Autodesk Inventor part; units mm, degrees
ref_plane "YZ Plane" through (0, 0, 0) normal (1, 0, 0) x (0, 1, 0)
ref_plane "XZ Plane" through (0, 0, 0) normal (0, 1, 0) x (-1, 0, 0)
ref_plane "XY Plane" through (0, 0, 0) normal (0, 0, 1) x (1, 0, 0)
sketch "Sketch1" plane through (0, 0, 0) normal (0, 0, 1) x (1, 0, 0)
  line L0 (-320.04, 0) -> (320.04, 0)
  line L1 (0, -340.36) -> (0, 86.36)
  line L2 (-228.6, 25.4) -> (228.6, 25.4)
  line L3 (-76.2, -279.4) -> (76.2, -279.4)
  line L4 (-228.6, 0) -> (-76.2, -279.4)
  line L5 (228.6, 0) -> (76.2, -279.4)
  line L6 (228.6, 0) -> (228.6, 25.4)
  line L7 (-228.6, 0) -> (-228.6, 25.4)
  point P0 (0, 0)
  point P1 (0, 25.4)
  point P2 (0, -279.4)
  point P3 (0, 25.4)
  dimension "d0" = 152.4
  dimension "d2" = 304.8
  dimension "d7" = 25.4
  dimension "d8" = 457.2
extrude "Extrusion1" add sketch "Sketch1" along normal mid plane 3.175
properties part number "electrical board back" material "ABS Plastic"
Could you check a few things on this model? Use its own coordinates, in mm. Give positions to 0.01 mm unless a question says otherwise; leave off trailing zeros. Loops run counter-clockwise (first coordinate to the right, second up) from the corner with the lowest first, then second, coordinate; pieces in that order, holes last. Notation, with made-up numbers: M 77.5,52.25 L 90.5,52.25 A18 cw 90.5,81.25 Z; hole C -28.5,17.25 d9. An arc over 180 degrees is marked long. Answer as a JSON object with one key per item and string values.
Q1. If I drill on probe 1 along X at (y, z) = (-263, 0.2); probe 2 along X at (y, z) = (-105, 0.15); probe 3 along Y at (x, z) = (199.5, -1.05), over which ranges is the centre line in solid material (lowest first)? Write a range as [from, to].
Values found:
{"probe 1": "x = [-85.15, 85.15]", "probe 2": "x = [-171.33, 171.33]", "probe 3": "y = [-53.35, 25.4]"}
Q2. Suppose I cut it at A-A, the plane x = 187.5. List the corners of the cut face in (y, z) for me, plus the area to 3 significant figures.
Values found:
{"outline": "M -75.35,-1.59 L 25.4,-1.59 L 25.4,1.59 L -75.35,1.59 Z", "area": "320 mm²"}
Q3. Suppose I cut it at B-B, the plane z = 1.1. List the corners of the cut face in (x, y) for me.
Values found:
{"outline": "M -228.6,0 L -76.2,-279.4 L 76.2,-279.4 L 228.6,0 L 228.6,25.4 L -228.6,25.4 Z"}
Q4. Suppose I cut it at C-C, the plane y = -196.5. List the corners of the cut face in (x, z) for me.
Values found:
{"outline": "M -121.42,-1.59 L 121.42,-1.59 L 121.42,1.59 L -121.42,1.59 Z"}
